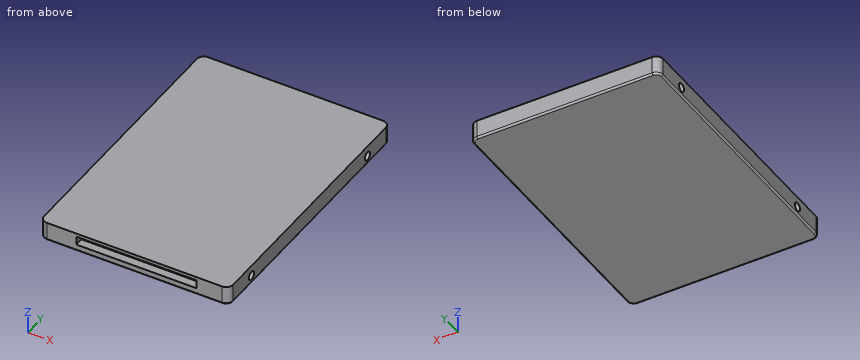
```python
from build123d import *

# Parameters (mm, degrees)
F0_W     = 69.85
F0_H     = 100.203
F1_DEPTH = 6.9088
F2_R     = 2.54
F3_R     = 1.5875
F4_DEPTH = 69.851
F5_R     = 0.635
F6_W     = 44.45
F6_H     = 3.175
F7_DEPTH = 3.175


with BuildPart() as f1:
    # F0 (on Top) → F1 (new body)
    with BuildSketch(Plane.XY):
        with Locations((34.925, 50.1015)):
            Rectangle(F0_W, F0_H)
    extrude(amount=F1_DEPTH)

    # F2
    f2_edges = [f1.edges().sort_by_distance(p)[0] for p in [
        (69.85, 0, 3.4544),
        (0, 0, 3.4544),
        (69.85, 100.203, 3.4544),
        (0, 100.203, 3.4544),
    ]]
    fillet(f2_edges, radius=F2_R)

    # F3 (on face) → F4 (cut, through all)
    with BuildSketch(Plane.YZ.offset(69.85)):
        with Locations((13.9954, 2.9972)):
            Circle(F3_R)
        with Locations((86.2076, 2.9972)):
            Circle(F3_R)
    extrude(amount=-F4_DEPTH, mode=Mode.SUBTRACT)

    # F5
    f5_edges = [f1.edges().sort_by_distance(p)[0] for p in [
        (69.85, 50.1015, 0),
        (69.106051, 0.743949, 0),
        (34.925, 0, 0),
        (0.743949, 0.743949, 0),
        (0, 50.1015, 0),
        (0.743949, 99.459051, 0),
        (34.925, 100.203, 0),
        (69.106051, 99.459051, 0),
    ]]
    fillet(f5_edges, radius=F5_R)

    # F6 (on face) → F7 (cut)
    with BuildSketch(Plane.XZ):
        with Locations((35.6616, 4.0513)):
            Rectangle(F6_W, F6_H)
    extrude(amount=-F7_DEPTH, mode=Mode.SUBTRACT)


solid = f1.part
```
For this review, take the finished solid that the model builds, in its own axes (mm). Coordinates: 2 decimals unless noted, no trailing zeros. Loops run counter-clockwise (first coordinate to the right, second up) from the corner with the lowest first, then second, coordinate; pieces in that order, holes last.
1. For line 1 (Y direction, x = 53.5, z = 2); line 2 (Y direction, x = 66, z = 0.5); line 3 (Y direction, x = 44, z = 2.25), list the stretches that pass through material, from the lowest coordinate up.
2. Insertion check: P1, Ø1.6, axis at y = 1.5, z = 4.5, coming from the +X side; P2, Ø1, axis at x = 36.5, z = 3.5, coming from the -Y side (3 decimals); P3, Ø1, axis at y = 1, z = 3.5, coming from the -X side. Each pin has a flat end and moves straight along its axis. Give the tip position at first contact, or say it passes through.
3. Add section A-A, the plane x = 17. Give the boundary of the cut face in (y, z) (1 decimal).
4. Add section B-B, the plane x = 59.5. Give the boundary of the cut face in (y, z) (1 decimal).
Result:
1. line 1: y = 0 to 12.76, 15.23 to 84.97, 87.44 to 100.2
1. line 2: y = 0.01 to 100.19
1. line 3: y = 0 to 12.59, 15.4 to 84.81, 87.61 to 100.2
2. P1: stops at x = 69.84
2. P2: stops at y = 3.175
2. P3: stops at x = 0.22
3. outline: (0, 0.6) arc R0.6 ccw to (0.6, 0) - (99.6, 0) arc R0.6 ccw to (100.2, 0.6) - (100.2, 6.9) - (0, 6.9) - (0, 5.6) - (3.2, 5.6) - (3.2, 2.5) - (0, 2.5) - close; hole circle Ø3.2 at (14, 3); hole circle Ø3.2 at (86.2, 3)
4. outline: (0, 0.6) arc R0.6 ccw to (0.6, 0) - (99.6, 0) arc R0.6 ccw to (100.2, 0.6) - (100.2, 6.9) - (0, 6.9) - close; hole circle Ø3.2 at (14, 3); hole circle Ø3.2 at (86.2, 3)
